Input: part model. Units: mm. Frame: model coordinates. Face numbers are marked on the shaded views. Coordinates: 2 decimals unless noted, no trailing zeros. Loops run counter-clockwise (first coordinate to the right, second up) from the corner with the lowest first, then second, coordinate; pieces in that order, holes last. Notation, with made-up numbers: (-38.5, -25) - (-11.5, -25) arc R7 cw to (-11.5, -17) - close; hole circle Ø8 at (78.5, 43). An arc over 180 degrees is marked (long way). Answer as CSV lines item,"result". Start each with the question number.
Autodesk Inventor part; units mm, degrees
ref_plane "YZ Plane" through (0, 0, 0) normal (1, 0, 0) x (0, 1, 0)
ref_plane "XZ Plane" through (0, 0, 0) normal (0, 1, 0) x (-1, 0, 0)
ref_plane "XY Plane" through (0, 0, 0) normal (0, 0, 1) x (1, 0, 0)
ref_plane "Work Plane1" through (-774.147, 14.6804, 0) normal (0, 0, -1) x (0.5974542, -0.801903, 0)
sketch "Sketch1" plane through (-774.147, 14.6804, 0) normal (0, 0, -1) x (0.5974542, -0.801903, 0)
  line L0 (58.7225, -26.2361) -> (-57.2775, -26.2361)
  line L1 (-57.2775, -26.2361) -> (-57.2775, 25.7639)
  line L2 (-57.2775, 25.7639) -> (58.7225, 25.7639)
  line L3 (58.7225, 25.7639) -> (58.7225, -26.2361)
  arc A0 (19.6988, -21.7639) -> (2.3103, -21.7639) centre (11.0046, -62.2541) ccw construction
  arc A1 (19.6988, -21.7639) -> (24.3194, -21.7639) centre (22.0091, -11.0045) ccw construction
  arc A2 (41.7079, -21.7639) -> (24.3194, -21.7639) centre (33.0137, -62.2541) ccw construction
  arc A3 (41.7079, -21.7639) -> (54.7775, -8.6943) centre (44.0182, -11.0045) ccw construction
  arc A4 (54.7775, 8.6943) -> (54.7775, -8.6943) centre (95.2678, 0) ccw construction
  arc A5 (54.7775, 8.6943) -> (41.7079, 21.7639) centre (44.0182, 11.0046) ccw construction
  arc A6 (24.3194, 21.7639) -> (41.7079, 21.7639) centre (33.0137, 62.2541) ccw construction
  arc A7 (24.3194, 21.7639) -> (19.6988, 21.7639) centre (22.0091, 11.0046) ccw construction
  arc A8 (2.3103, 21.7639) -> (19.6988, 21.7639) centre (11.0046, 62.2541) ccw construction
  arc A9 (2.3103, 21.7639) -> (-2.3103, 21.7639) centre (0, 11.0046) ccw construction
  arc A10 (-19.6988, 21.7639) -> (-2.3103, 21.7639) centre (-11.0045, 62.2541) ccw construction
  arc A11 (-19.6988, 21.7639) -> (-24.3194, 21.7639) centre (-22.0091, 11.0046) ccw construction
  arc A12 (-41.7079, 21.7639) -> (-24.3194, 21.7639) centre (-33.0136, 62.2541) ccw construction
  arc A13 (-41.7079, 21.7639) -> (-54.7775, 8.6943) centre (-44.0182, 11.0046) ccw construction
  arc A14 (-54.7775, -8.6943) -> (-54.7775, 8.6943) centre (-95.2678, 0) ccw construction
  arc A15 (-54.7775, -8.6943) -> (-41.7079, -21.7639) centre (-44.0182, -11.0045) ccw construction
  arc A16 (-24.3194, -21.7639) -> (-41.7079, -21.7639) centre (-33.0136, -62.2541) ccw construction
  arc A17 (-24.3194, -21.7639) -> (-19.6988, -21.7639) centre (-22.0091, -11.0045) ccw construction
  arc A18 (-2.3103, -21.7639) -> (-19.6988, -21.7639) centre (-11.0045, -62.2541) ccw construction
  arc A19 (-2.3103, -21.7639) -> (2.3103, -21.7639) centre (0, -11.0045) ccw construction
  line L4 (159.874, 0.748) -> (161.144, 0.748) construction
  line L5 (161.144, 0.748) -> (161.144, -3.697) construction
  line L6 (159.874, -3.697) -> (161.144, -3.697) construction
  line L7 (159.874, -3.697) -> (159.874, 0.748) construction
  line L8 (63.7225, -31.2361) -> (-62.2775, -31.2361)
  line L9 (-62.2775, -31.2361) -> (-62.2775, 30.7639)
  line L10 (-62.2775, 30.7639) -> (63.7225, 30.7639)
  line L11 (63.7225, 30.7639) -> (63.7225, -31.2361)
  line L12 (58.7225, -26.2361) -> (63.7225, -26.2361)
  line L13 (-57.2775, -26.2361) -> (-62.2775, -26.2361)
  line L14 (-57.2775, 25.7639) -> (-62.2775, 25.7639)
  line L15 (58.7225, 25.7639) -> (63.7225, 25.7639)
  point P0 (474.2897, -612.02)
  dimension "d0" = 116
  dimension "d1" = 52
  dimension "d2" = 2.5
  dimension "d3" = 4
  dimension "d4" = 5
extrude "Extrusion1" add sketch "Sketch1" against normal blind 47 contours L12 L11 L8 L9 L13 L0 | L13 L9 L14 L1 | L2 L14 L9 L10 L11 L15
sketch "Sketch2" plane through (-774.147, 14.6804, 47) normal (0, 0, 1) x (0.5974542, -0.801903, 0)
  line L0 (-62.2775, -30.7639) -> (63.7225, -30.7639)
  line L1 (63.7225, 31.2361) -> (-62.2775, 31.2361)
  line L2 (63.7225, -30.7639) -> (-62.2775, -30.7639)
  line L3 (-62.2775, -30.7639) -> (-62.2775, 31.2361)
  line L4 (-62.2775, 31.2361) -> (63.7225, 31.2361)
  line L5 (63.7225, 31.2361) -> (63.7225, -30.7639)
  point P0 (474.2897, 612.02)
  point P1 (-62.2775, -30.7639)
  point P2 (63.7225, 31.2361)
extrude "Extrusion2" add sketch "Sketch2" along normal blind 3
fillet "Fillet1" radius 1.5875 6 edges at (-711.0274, -17.7567, 25) (-786.3067, 83.283, 25) (-760.7454, -54.7989, 25) (-756.7359, -51.8116, 23.5) (-715.037, -20.744, 23.5) (-836.0247, 46.2409, 25)
ref_plane "Work Plane2" through (-841.5049, -36.3773, 0) normal (0, 0, 1) x (0.6694225, -0.7428819, 0)
sketch "Sketch3" plane through (-841.5049, -36.3773, 0) normal (0, 0, 1) x (0.6694225, -0.7428819, 0)
  line L0 (-50.362, 120.9615) -> (71.931, 109.5419)
  line L1 (66.1667, 47.8105) -> (-56.1263, 59.23)
  line L2 (73.3641, 107.8137) -> (73.1944, 105.9966)
  line L3 (-57.5594, 60.9582) -> (-52.0902, 119.5284)
  circle A0 centre (-39.2118, 52.5485) radius 2.15
  circle A1 centre (48.3075, 44.3761) radius 2.15
  line L4 (68.0646, 51.0606) -> (67.8949, 49.2435)
  arc A2 (-44.0243, 54.1752) -> (-34.1813, 53.2561) centre (-39.2118, 52.5485) ccw
  line L5 (40.7824, 50.1808) -> (48.7798, 49.434)
  arc A3 (-44.0243, 54.1752) -> (-46.7369, 58.3532) centre (-47.0321, 55.192) ccw
  arc A4 (-30.7421, 56.8597) -> (-34.1813, 53.2561) centre (-31.0373, 53.6984) ccw
  arc A5 (43.495, 46.0028) -> (53.338, 45.0837) centre (48.3075, 44.3761) ccw
  arc A6 (43.495, 46.0028) -> (40.7824, 50.1808) centre (40.4872, 47.0196) ccw
  arc A7 (43.495, 46.0028) -> (40.7824, 50.1808) centre (40.4872, 47.0196) ccw
  line L6 (66.1667, 47.8105) -> (40.7824, 50.1808)
  arc A8 (43.495, 46.0028) -> (40.7824, 50.1808) centre (40.4872, 47.0196) ccw
  line L7 (48.3075, 44.3761) -> (48.6282, 47.8105)
  arc A9 (56.7772, 48.6873) -> (53.338, 45.0837) centre (56.482, 45.526) ccw
  line L8 (-54.8248, 90.2433) -> (-8.2036, 85.8899) construction
  line L9 (71.931, 109.5419) -> (-50.362, 120.9615)
  circle A10 centre (-32.5028, 124.3959) radius 2.15
  circle A11 centre (55.0165, 116.2235) radius 2.15
  line L10 (73.1944, 105.9966) -> (73.3641, 107.8137)
  arc A12 (-27.6903, 122.7691) -> (-37.5332, 123.6882) centre (-32.5028, 124.3959) ccw
  line L11 (46.5468, 111.9123) -> (54.5442, 111.1655)
  arc A13 (-40.9725, 120.0847) -> (-37.5332, 123.6882) centre (-40.6773, 123.2459) ccw
  arc A14 (-27.6903, 122.7691) -> (-24.9777, 118.5911) centre (-24.6825, 121.7524) ccw
  arc A15 (59.829, 114.5967) -> (49.986, 115.5158) centre (55.0165, 116.2235) ccw
  arc A16 (46.5468, 111.9123) -> (49.986, 115.5158) centre (46.842, 115.0735) ccw
  arc A17 (46.5468, 111.9123) -> (49.986, 115.5158) centre (46.842, 115.0735) ccw
  line L12 (71.931, 109.5419) -> (46.5468, 111.9123)
  arc A18 (46.5468, 111.9123) -> (49.986, 115.5158) centre (46.842, 115.0735) ccw
  line L13 (55.0165, 116.2235) -> (54.6958, 112.7891)
  arc A19 (59.829, 114.5967) -> (62.5416, 110.4187) centre (62.8368, 113.58) ccw
  point P0 (536.2982, 649.4905)
  point P1 (73.2792, 106.9052)
  point P2 (48.7798, 49.434)
  point P3 (54.5442, 111.1655)
  point P4 (-40.9725, 120.0847)
  point P5 (-24.9777, 118.5911)
  point P6 (49.986, 115.5158)
  point P7 (46.5468, 111.9123)
  point P8 (62.5416, 110.4187)
  point P9 (43.495, 46.0028)
  point P10 (56.7772, 48.6873)
  point P11 (40.7824, 50.1808)
  point P12 (-30.7421, 56.8597)
  point P13 (-46.7369, 58.3532)
  dimension "d16" = 4.3
  dimension "d18" = 4.3
  dimension "d20" = 19.05
  dimension "d21" = 19.05
  dimension "d24" = 5.08
  dimension "d25" = 3.175
  dimension "d26" = 3.175
  dimension "d27" = 3.175
  dimension "d28" = 5.08
  dimension "d29" = 3.175
  dimension "d30" = 3.175
extrude "Extrusion3" add sketch "Sketch3" along normal blind 3
properties part number "Battery_Holder"
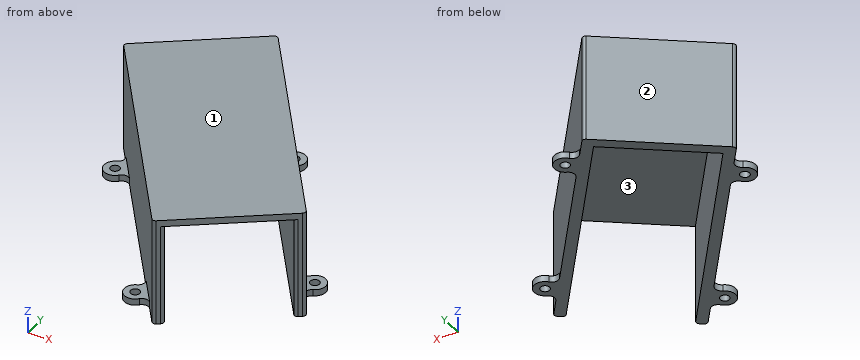
Item 1: Section query A-A, the plane z = 17. Output: boundary loops of the cut face in (x, y) (1 decimal).
Item 2: Section query C-C, the plane x = -724.5. Output: boundary loops of the cut face in (y, z).
Item 3: Contact query for flat-ended pins moving along their axis: P1, Ø2, axis at y = -6, z = 8.5, coming from the -X side; P2, Ø8, axis at y = -31.5, z = 10.5, coming from the -X side; P3, Ø12, axis at x = -757.5, z = 8, coming from the +Y side; P4, Ø15.5, axis at x = -777.5, y = -38, coming from the +Z side. Output: stop coordinate, or through.
Item 4: Section query B-B, the plane y = 52.5. Output: boundary loops of the cut face in (x, z), and give its area (3 significant figures).
Item 5: Draft query along X for the marked faces 1, 2 and 3. Return one class per face: pulls with the +X half, pulls with the -X half, needs draft (parallel to the pull), parting line crosses it, or undercut.
Item 6: Section query D-D, the plane x = -738. Output: boundary loops of the cut face in (y, z).
Item 7: Material intervals for probe 1 along Z at (x, y) = (-778, 2); probe 2 along X at (y, z) = (9.5, 27.5); probe 3 along Y at (x, z) = (-798.5, 44.5), sorted ascending.
Response values:
1,outline,"(-835.1, 45) - (-761.7, -53.5) arc R1.6 ccw to (-759.5, -53.9) - (-758, -52.8) arc R1.6 ccw to (-757.7, -50.5) - (-829, 45.2) - (-787.3, 76.3) - (-716, -19.5) arc R1.6 ccw to (-713.8, -19.8) - (-712.3, -18.7) arc R1.6 ccw to (-712, -16.5) - (-785.4, 82) arc R1.6 ccw to (-787.6, 82.3) - (-834.8, 47.2) arc R1.6 ccw to start"
2,outline,"(-27.79, 47) - (-8.04, 47) - (-8.04, 0) - (2.69, 0) - (2.69, 3) - (0.33, 3) - (0.33, 50) - (-27.79, 50) - close"
3,P1,"stops at x = -797.85"
3,P2,"stops at x = -781.08"
3,P3,"stops at y = 52.67"
3,P4,"stops at z = 50"
4,outline,"(-827.62, 0) - (-819.25, 0) - (-819.25, 47) - (-769.61, 47) - (-769.61, 0) - (-763.37, 0) - (-763.37, 50) - (-827.62, 50) - close"
4,area,"879 mm²"
5,face 1,"needs draft"
5,face 2,"pulls with the -X half"
5,face 3,"undercut"
6,outline,"(-37.85, 47) - (10.08, 47) - (10.08, 0) - (18.45, 0) - (18.45, 50) - (-37.85, 50) - close"
7,probe 1,"z = 47 to 50"
7,probe 2,"x = -808.65 to -802.42, -737.57 to -731.33"
7,probe 3,"y = -4.12 to 4.24, 67.96 to 74.2"
